The figure shows three views and two pictorial views of one solid part (mm, origin at its lowest corner). Answer the questions. Coordinates: 2 decimals unless noted, no trailing zeros. Order: outer loops, then holes, each group sorted by start corner. A loop starts at its lowest first (then second) coordinate and runs counter-clockwise, first axis right, second up. Notation, with made-up numbers: M 43,-37.75 L 56,-37.75 A10 cw 56,-20.75 Z; hole C -14,80.25 d6. An arc over 180 degrees is marked long. Use a Markdown table: item, result.
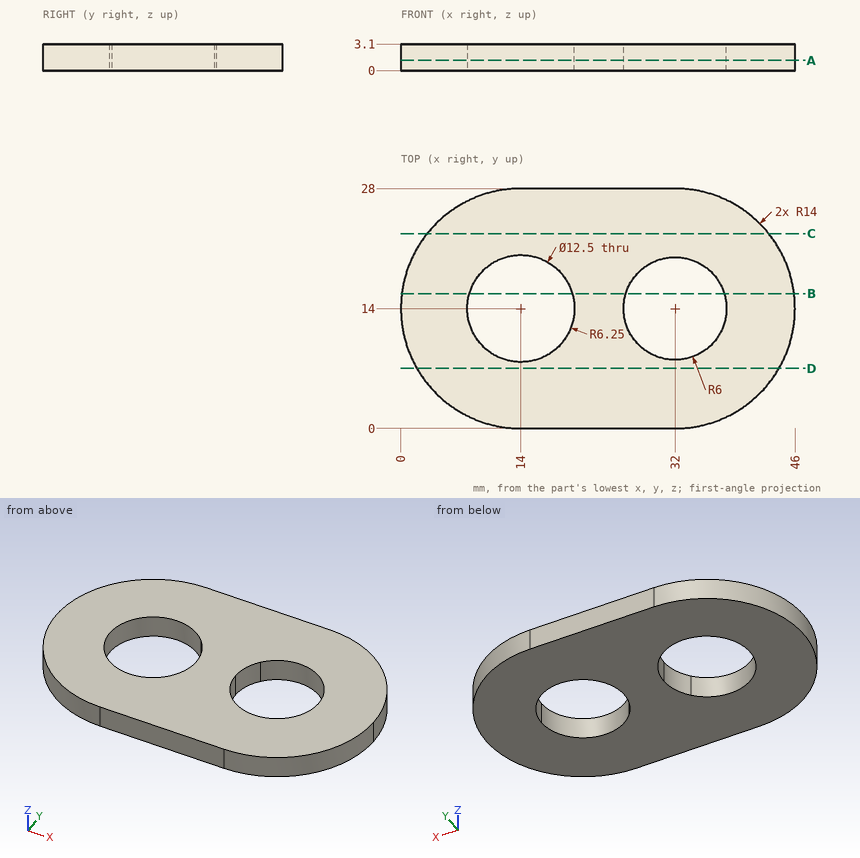
1. Section D-D on y = 7 is taken. Determine the outline of the cut face in (x, z), then the cut area to 3 significant figures.
Answers below:
| item | result |
|---|---|
| outline | M 1.88,0 L 44.12,0 L 44.12,3.1 L 1.88,3.1 Z |
| area | 131 mm² |
2. Section C-C on y = 22.75 is taken. Determine the outline of the cut face in (x, z), then the cut area to 3 significant figures.
Answers below:
| item | result |
|---|---|
| outline | M 3.07,0 L 42.93,0 L 42.93,3.1 L 3.07,3.1 Z |
| area | 124 mm² |
3. A flat-ended cylindrical pin translates along its axis: P1, Ø5, axis at x = 16.5, y = 11, coming from the -Z side. Find the tip coordinate at first contact, or state that the pin passes through.
Answers below:
| item | result |
|---|---|
| P1 | z = 0 |
4. Find the intervals of material crossed by probe 1 along X at (y, z) = (14, 1.2); probe 2 along Y at (x, z) = (14, 1.05); probe 3 along X at (y, z) = (15.5, 0.65), in increasing order.
Answers below:
| item | result |
|---|---|
| probe 1 | 0 to 7.75, 20.25 to 26, 38 to 46 |
| probe 2 | 0 to 7.75, 20.25 to 28 |
| probe 3 | 0.08 to 7.93, 20.07 to 26.19, 37.81 to 45.92 |
5. Section A-A on z = 1.2 is taken. Determine the outline of the cut face in (x, y), then the cut area to 3 significant figures.
Answers below:
| item | result |
|---|---|
| outline | M 14,0 L 32,0 A14 ccw 32,28 L 14,28 A14 ccw Z; hole C 14,14 d12.5; hole C 32,14 d12 |
| area | 884 mm² |
6. Section B-B on y = 15.75 is taken. Determine the outline of the cut face in (x, z), then the cut area to 3 significant figures.
Answers below:
| item | result |
|---|---|
| outline | M 0.11,0 L 8,0 L 8,3.1 L 0.11,3.1 Z; M 20,0 L 26.26,0 L 26.26,3.1 L 20,3.1 Z; M 37.74,0 L 45.89,0 L 45.89,3.1 L 37.74,3.1 Z |
| area | 69.1 mm² |
